Geometry: see drawing. Coordinates: mm, zero at the bounding-box minimum. Give positions to 0.01 mm unless a question says otherwise; leave off trailing zeros. Order: outer loops, then holes, each group sorted by start corner. A loop starts at its lowest first (then second) coordinate and runs counter-clockwise, first axis right, second up. Notation, with made-up numbers: (44, -10) - (86, -10) arc R22 cw to (86, 16) - close; hole circle Ø4 at (-2.5, -12.5). An arc over 180 degrees is marked (long way). Put each result on its own line as item: value. Start each with the question number.
1. Section C-C on z = 3.75. Return the cut outline in (x, y).
2. Mould query, pull axis X, two halves, no side actions, for the marked faces 1 and 2. Classes: pulls with the +X half, pulls with the -X half, needs draft (parallel to the pull), parting line crosses it, or undercut.
3. First-contact query: P1, Ø4, axis at x = 123, y = 35, coming from the +Z side. Flat tip, straight axial feed; report the tip coordinate or a pass-through.
4. Section B-B on y = 38.5. Return the cut outline in (x, z).
5. Ray query, line 1 along Y through (x, z) = (112, 8.75); line 2 along X through (y, z) = (18, 6); line 3 along Y through (x, z) = (15, 4.25). Return the intervals inside material, ascending. Write a range as from..to.
6. Section A-A on x = 88. Return the cut outline in (y, z).
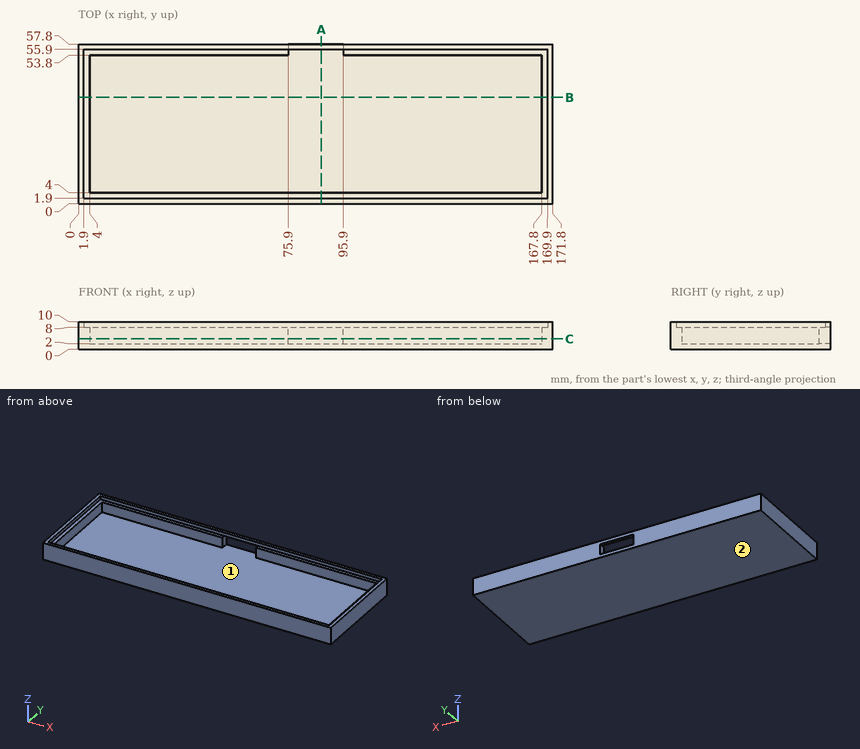
Resolved:
1. outline: (0, 0) - (171.8, 0) - (171.8, 57.8) - (95.9, 57.8) - (95.9, 53.8) - (167.8, 53.8) - (167.8, 4) - (4, 4) - (4, 53.8) - (75.9, 53.8) - (75.9, 57.8) - (0, 57.8) - close
2. face 1: undercut
2. face 2: needs draft
3. P1: z = 2
4. outline: (0, 0) - (171.8, 0) - (171.8, 10) - (169.9, 10) - (169.9, 8) - (167.8, 8) - (167.8, 2) - (4, 2) - (4, 8) - (1.9, 8) - (1.9, 10) - (0, 10) - close
5. line 1: 0..1.9, 55.9..57.8
5. line 2: 0..4, 167.8..171.8
5. line 3: 0..4, 53.8..57.8
6. outline: (0, 0) - (57.8, 0) - (57.8, 2) - (4, 2) - (4, 8) - (1.9, 8) - (1.9, 10) - (0, 10) - close; (55.9, 8) - (57.8, 8) - (57.8, 10) - (55.9, 10) - close
